The drawing under review shows one solid part. Ordinate dimensions are in mm from its lowest x, y, z. Coordinates: 2 decimals unless noted, no trailing zeros. Write each loop counter-clockwise with the first axis right and the second up, starting at its lowest first coordinate (ties: lowest second). Pieces come first, ordered by that corner, then holes.
Q1. Mouldability with a two-part tool opening along X and no side actions: class the marked faces 1, 2, 3 and 4 as pulls with the +X half, pulls with the -X half, needs draft (parallel to the pull), parting line crosses it, or undercut.
Q2. Insertion check: pin 1 (4 mm diameter, centred on x = 26.5, y = 3.5, fed in from +Z); pin 2 (1 mm diameter, centred on y = 9, z = 3, fed in from +X). Each pin has a flat end and moves straight along its axis. Give the tip position at first contact, or say it passes through.
Q3. Take a section at A-A (y = 3.25). Give the boundary of the cut face in (x, z), and give its area (3 significant figures).
Q4. For probe 1 along X at (y, z) = (10.75, 6.25); probe 2 along Y at (x, z) = (3.55, 4.5); probe 3 along Z at (x, y) = (19.5, 9.75), list the stretches that pass through material, from the lowest coordinate up.
Q5. Take a section at B-B (z = 4.5). Give the boundary of the cut face in (x, y), and give its area (3 significant figures).
Q6. Take a section at D-D (y = 12.25). Give the boundary of the cut face in (x, z), and give its area (3 significant figures).
Q7. Take a section at C-C (z = 6.5). Give the boundary of the cut face in (x, y), and give its area (3 significant figures).
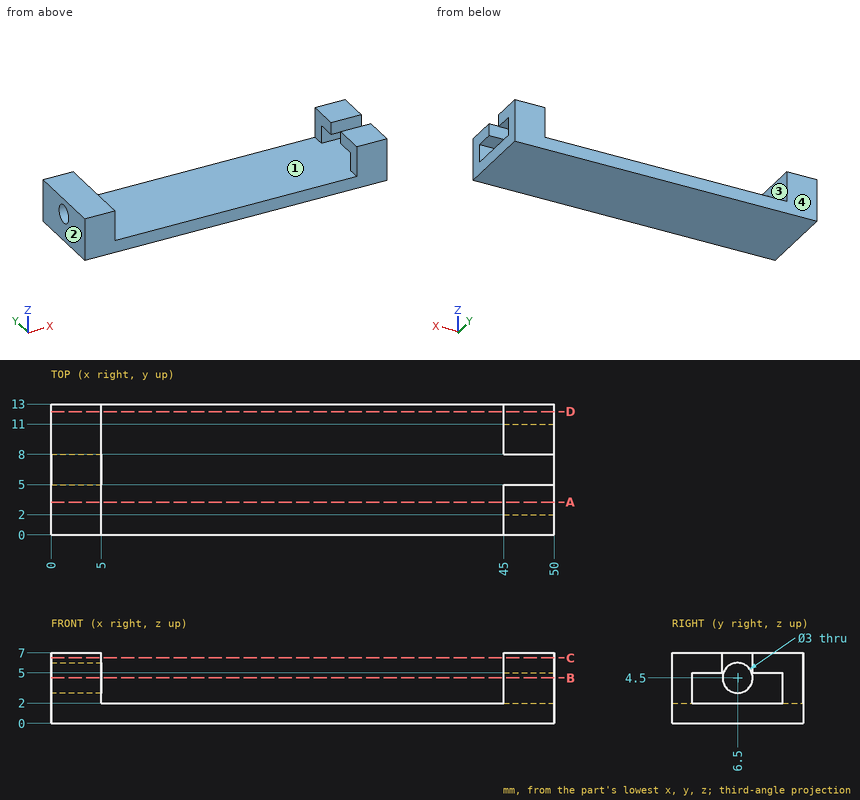
Response:
1. face 1: undercut
1. face 2: pulls with the -X half
1. face 3: undercut
1. face 4: needs draft
2. pin 1: stops at z = 2
2. pin 2: stops at x = 5
3. outline: (0, 0) - (50, 0) - (50, 2) - (5, 2) - (5, 7) - (0, 7) - close; (45, 5) - (50, 5) - (50, 7) - (45, 7) - close
3. area: 135 mm2
4. probe 1: x = 0 to 5, 45 to 50
4. probe 2: y = 0 to 5, 8 to 13
4. probe 3: z = 0 to 2
5. outline: (0, 0) - (5, 0) - (5, 5) - (0, 5) - close; (0, 8) - (5, 8) - (5, 13) - (0, 13) - close; (45, 0) - (50, 0) - (50, 2) - (45, 2) - close; (45, 11) - (50, 11) - (50, 13) - (45, 13) - close
5. area: 70.0 mm2
6. outline: (0, 0) - (50, 0) - (50, 7) - (45, 7) - (45, 2) - (5, 2) - (5, 7) - (0, 7) - close
6. area: 150 mm2
7. outline: (0, 0) - (5, 0) - (5, 13) - (0, 13) - close; (45, 0) - (50, 0) - (50, 5) - (45, 5) - close; (45, 8) - (50, 8) - (50, 13) - (45, 13) - close
7. area: 115 mm2
